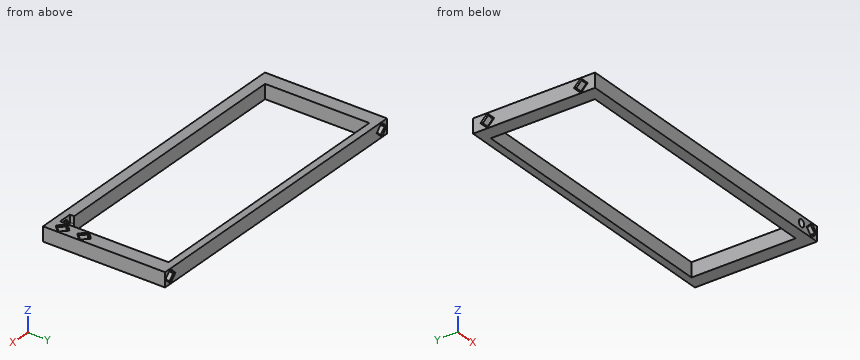
from build123d import *

# Parameters (mm, degrees)
SKETCH1_W                              = 178.0009902
SKETCH1_H                              = 72.120000116
SKETCH1_W_2                            = 161.067656866
SKETCH1_H_2                            = 61.536666783
BOSS_EXTRUDE1_DEPTH                    = 8.466666667
CUT_EXTRUDE1_DEPTH                     = 5.08
CUT_EXTRUDE2_DEPTH                     = 5.08
CUT_EXTRUDE3_DEPTH                     = 5.08
CUT_EXTRUDE4_DEPTH                     = 5.08
CHAMFER1_SIZE                          = 0.635
CUT_EXTRUDE5_DEPTH                     = 2.54
F_18_0_1695_DIAMETER_HOLE1_D           = 4.3053
F_18_0_1695_DIAMETER_HOLE1_DEPTH       = 3.81
F_18_0_1695_DIAMETER_HOLE1_CSINK_D     = 5.5753
F_18_0_1695_DIAMETER_HOLE1_CSINK_ANGLE = 90


with BuildPart() as part:
    # Sketch1 → Boss-Extrude1 (new body)
    with BuildSketch(Plane.XY):
        Rectangle(SKETCH1_W, SKETCH1_H)
        with Locations((0, 1.058333334)):
            Rectangle(SKETCH1_W_2, SKETCH1_H_2, mode=Mode.SUBTRACT)
    extrude(amount=BOSS_EXTRUDE1_DEPTH)

    # Sketch2 → Cut-Extrude1 (cut)
    with BuildSketch(Plane(origin=(0, 36.060000058, 0), x_dir=(1, 0, 0), z_dir=(0, 1, 0))):
        Polygon((-87.942161767, -4.233333333), (-84.767161767, -1.058333333), (-81.592161767, -4.233333333), (-84.767161767, -7.408333333), align=None)
        Polygon((81.592161767, -4.233333333), (84.767161767, -1.058333333), (87.942161767, -4.233333333), (84.767161767, -7.408333333), align=None)
    extrude(amount=-CUT_EXTRUDE1_DEPTH, mode=Mode.SUBTRACT)

    # Sketch3 → Cut-Extrude2 (cut)
    with BuildSketch(Plane.XY.offset(8.466666667)):
        Polygon((81.592161767, -27.593333392), (84.767161767, -24.418333392), (87.942161767, -27.593333392), (84.767161767, -30.768333392), align=None)
        Polygon((84.767161767, -11.718333392), (87.942161767, -14.893333392), (84.767161767, -18.068333392), (81.592161767, -14.893333392), align=None)
    extrude(amount=-CUT_EXTRUDE2_DEPTH, mode=Mode.SUBTRACT)

    # Sketch4 → Cut-Extrude3 (cut)
    with BuildSketch(Plane.ZY.offset(89.0004951)):
        Polygon((1.058333333, 27.593333392), (4.233333333, 30.768333392), (7.408333333, 27.593333392), (4.233333333, 24.418333392), align=None)
        Polygon((1.058333333, -27.593333392), (4.233333333, -24.418333392), (7.408333333, -27.593333392), (4.233333333, -30.768333392), align=None)
    extrude(amount=-CUT_EXTRUDE3_DEPTH, mode=Mode.SUBTRACT)

    # Sketch5 → Cut-Extrude4 (cut)
    with BuildSketch(Plane.XZ.offset(36.060000058)):
        Polygon((81.592161767, 4.233333333), (84.767161767, 7.408333333), (87.942161767, 4.233333333), (84.767161767, 1.058333333), align=None)
    extrude(amount=-CUT_EXTRUDE4_DEPTH, mode=Mode.SUBTRACT)

    # Chamfer1
    chamfer1_edges = [part.edges().sort_by_distance(p)[0] for p in [
        (83.179661767, -30.980000058, 2.645833333),
        (83.179661767, -30.980000058, 5.820833333),
        (86.354661767, -30.980000058, 5.820833333),
        (86.354661767, -30.980000058, 2.645833333),
        (83.179661767, -36.060000058, 2.645833333),
        (86.354661767, -36.060000058, 2.645833333),
        (86.354661767, -36.060000058, 5.820833333),
        (83.179661767, -36.060000058, 5.820833333),
        (-86.354661767, 30.980000058, 5.820833333),
        (-86.354661767, 30.980000058, 2.645833333),
        (-83.179661767, 30.980000058, 2.645833333),
        (-83.179661767, 30.980000058, 5.820833333),
        (-86.354661767, 36.060000058, 5.820833333),
        (-83.179661767, 36.060000058, 5.820833333),
        (-83.179661767, 36.060000058, 2.645833333),
        (-86.354661767, 36.060000058, 2.645833333),
        (83.179661767, 30.980000058, 5.820833333),
        (83.179661767, 30.980000058, 2.645833333),
        (86.354661767, 30.980000058, 2.645833333),
        (86.354661767, 30.980000058, 5.820833333),
        (83.179661767, 36.060000058, 5.820833333),
        (86.354661767, 36.060000058, 5.820833333),
        (86.354661767, 36.060000058, 2.645833333),
        (83.179661767, 36.060000058, 2.645833333),
        (83.179661767, -29.180833392, 3.386666667),
        (83.179661767, -26.005833392, 3.386666667),
        (86.354661767, -26.005833392, 3.386666667),
        (86.354661767, -29.180833392, 3.386666667),
        (83.179661767, -29.180833392, 8.466666667),
        (86.354661767, -29.180833392, 8.466666667),
        (86.354661767, -26.005833392, 8.466666667),
        (83.179661767, -26.005833392, 8.466666667),
        (83.179661767, -13.305833392, 3.386666667),
        (86.354661767, -13.305833392, 3.386666667),
        (86.354661767, -16.480833392, 3.386666667),
        (83.179661767, -16.480833392, 3.386666667),
        (83.179661767, -13.305833392, 8.466666667),
        (83.179661767, -16.480833392, 8.466666667),
        (86.354661767, -16.480833392, 8.466666667),
        (86.354661767, -13.305833392, 8.466666667),
        (-83.9204951, 26.005833392, 2.645833333),
        (-83.9204951, 29.180833392, 2.645833333),
        (-83.9204951, 29.180833392, 5.820833333),
        (-83.9204951, 26.005833392, 5.820833333),
        (-89.0004951, 26.005833392, 2.645833333),
        (-89.0004951, 26.005833392, 5.820833333),
        (-89.0004951, 29.180833392, 5.820833333),
        (-89.0004951, 29.180833392, 2.645833333),
        (-83.9204951, -29.180833392, 2.645833333),
        (-83.9204951, -26.005833392, 2.645833333),
        (-83.9204951, -26.005833392, 5.820833333),
        (-83.9204951, -29.180833392, 5.820833333),
        (-89.0004951, -29.180833392, 2.645833333),
        (-89.0004951, -29.180833392, 5.820833333),
        (-89.0004951, -26.005833392, 5.820833333),
        (-89.0004951, -26.005833392, 2.645833333),
    ]]
    chamfer(chamfer1_edges, length=CHAMFER1_SIZE)

    # Sketch6 → Cut-Extrude5 (cut)
    with BuildSketch(Plane(origin=(0, -29.710000058, 0), x_dir=(1, 0, 0), z_dir=(0, 1, 0))):
        with BuildLine():
            Line((72.659828433, -4.233333249), (72.659828433, -8.466666667))
            Line((72.659828433, -8.466666667), (80.533828433, -8.466666667))
            Line((80.533828433, -8.466666667), (80.533828433, -4.233333249))
            ThreePointArc((80.533828433, -4.233333249), (76.596828433, -0.296333249), (72.659828433, -4.233333249))
        make_face()
    extrude(amount=-CUT_EXTRUDE5_DEPTH, mode=Mode.SUBTRACT)

    # #18 (0.1695) Diameter Hole1
    with Locations(Plane(origin=(0, -32.250000058, 0), x_dir=(1, 0, 0), z_dir=(0, 1, 0))):
        with Locations((76.596828433, -4.233333249)):
            CounterSinkHole(F_18_0_1695_DIAMETER_HOLE1_D / 2, F_18_0_1695_DIAMETER_HOLE1_CSINK_D / 2, depth=F_18_0_1695_DIAMETER_HOLE1_DEPTH, counter_sink_angle=F_18_0_1695_DIAMETER_HOLE1_CSINK_ANGLE)


solid = part.part
Read the model definition and answer for the solid it produces. Units are mm, in the model's axes. Coordinates: 2 decimals unless noted, no trailing zeros. Loops run counter-clockwise (first coordinate to the right, second up) from the corner with the lowest first, then second, coordinate; pieces in that order, holes last. Notation, with made-up numbers: (-13.75, -5.75) -> (3.25, -5.75) arc R31 ccw to (3.25, 31.25) -> close; hole circle Ø1 at (51.5, 35). An arc over 180 degrees is marked (long way). Answer in a Markdown table with one row per item.
Item 1: Straight lines are drawn through the part: line 1 along Y through (x, z) = (-67, 2); line 2 along X through (y, z) = (18.5, 2); line 3 along X through (y, z) = (-27, 3.5). For each, find the intervals that lie inside material, in ascending order. Write a range as [from, to].
Returned:
| item | result |
|---|---|
| line 1 | y = [-36.06, -29.71], [31.83, 36.06] |
| line 2 | x = [-89, -80.53], [80.53, 89] |
| line 3 | x = [-83.92, -80.53], [80.53, 82.92], [86.61, 89] |
Item 2: Each of these flat-tipped pins is pushed along its axis until it touches: P1, Ø1.4, axis at x = 84, y = -15.5, coming from the +Z side; P2, Ø2.5, axis at x = 84.5, y = -26.5, coming from the +Z side; P3, Ø3.5, axis at y = -28, z = 5, coming from the -X side. Where does it stop, or does it pass through?
Returned:
| item | result |
|---|---|
| P1 | stops at z = 3.45 |
| P2 | stops at z = 3.99 |
| P3 | stops at x = -88.7 |
Item 3: A cutting plane is placed at B-B on y = 1. Determine the outline of the cut face in (x, z), plus the area to 3 significant figures.
Returned:
| item | result |
|---|---|
| outline | (-89, 0) -> (-80.53, 0) -> (-80.53, 8.47) -> (-89, 8.47) -> close; (80.53, 0) -> (89, 0) -> (89, 8.47) -> (80.53, 8.47) -> close |
| area | 143 mm^2 |
Item 4: A cutting plane is placed at A-A on x = 45. Determine the outline of the cut face in (y, z).
Returned:
| item | result |
|---|---|
| outline | (-36.06, 0) -> (-29.71, 0) -> (-29.71, 8.47) -> (-36.06, 8.47) -> close; (31.83, 0) -> (36.06, 0) -> (36.06, 8.47) -> (31.83, 8.47) -> close |
